Build history of the part. All positions in model axes, mm. Round coordinates to 2 decimals unless told otherwise and drop trailing zeros. Order: outer loops, then holes, each group sorted by start corner. A loop starts at its lowest first (then second) coordinate and runs counter-clockwise, first axis right, second up. Notation, with made-up numbers: M 16,54.25 L 70,54.25 A26 ccw 70,82.25 Z; hole C 87,20.5 d6. An arc over 180 degrees is marked long. Use CSV: the item, a comma, the result in double quotes.
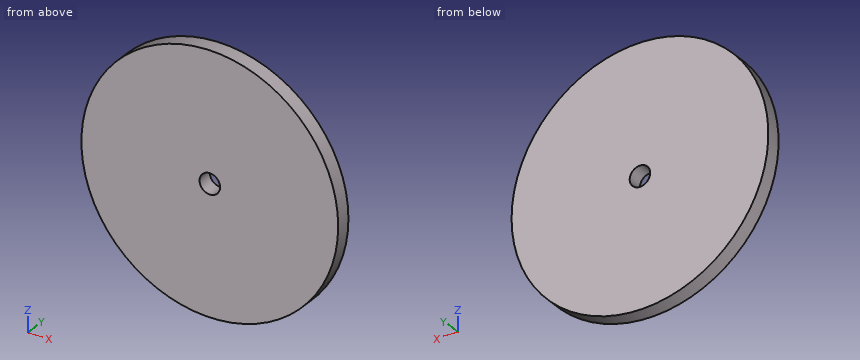
Autodesk Inventor part; units mm, degrees
ref_plane "YZ Plane" through (0, 0, 0) normal (1, 0, 0) x (0, 1, 0)
ref_plane "XZ Plane" through (0, 0, 0) normal (0, 1, 0) x (-1, 0, 0)
ref_plane "XY Plane" through (0, 0, 0) normal (0, 0, 1) x (1, 0, 0)
sketch "スケッチ1" plane through (0, 0, 0) normal (0, 1, 0) x (-1, 0, 0)
  circle A0 centre (0, 0) radius 25
  dimension "d0" = 50
extrude "押し出し1" add sketch "スケッチ1" along normal blind 6
sketch "スケッチ2" plane through (0, 6, 0) normal (0, 1, 0) x (1, 0, 0)
  circle A0 centre (0, 0) radius 4
  dimension "d3" = 8
extrude "押し出し2" cut sketch "スケッチ2" against normal blind 6
sketch "スケッチ3" plane through (0, 0, 0) normal (0, -1, 0) x (1, 0, 0)
  circle A0 centre (0, 0) radius 45
  circle A1 centre (0, 0) radius 4
  circle A2 centre (0, 0) radius 25
  dimension "d6" = 90
  dimension "d7" = 50
extrude "押し出し3" add sketch "スケッチ3" against normal blind 6 contours A0
sketch "スケッチ4" plane through (0, 6, 0) normal (0, 1, 0) x (1, 0, 0)
  circle A0 centre (0, 0) radius 45
  circle A1 centre (0, 0) radius 50
  dimension "d10" = 90
  dimension "d11" = 100
extrude "押し出し4" add sketch "スケッチ4" against normal blind 6
properties part number "NHK_t0_3"
(1) Drop flat-ended pins along their axis: pin 1 (3 mm diameter, centred on x = -20, y = 1.5, fed in from -Z); pin 2 (2 mm diameter, centred on y = 3.5, z = -30, fed in from +X); pin 3 (1.5 mm diameter, centred on x = 14, y = 5, fed in from +Z). Give the stop position or say it passes through.
Answer block:
pin 1,"stops at z = -46.45"
pin 2,"stops at x = 40.73"
pin 3,"stops at z = 48.21"
(2) Cut at B-B, the plane x = 0. Give the cut face in (y, z).
Answer block:
outline,"M 0,-50 L 6,-50 L 6,-4 L 0,-4 Z; M 0,4 L 6,4 L 6,50 L 0,50 Z"
(3) Wall check: line 1 (Z direction, x = 0, y = 2.3); line 2 (X direction, y = 5.5, z = 41.5). Give the ranges that are in metal, low to high. Write a range as from..to.
Answer block:
line 1,"z = -50..-4, 4..50"
line 2,"x = -27.89..27.89"
(4) Cut at A-A, the plane z = 0. Give the cut face in (x, y).
Answer block:
outline,"M -50,0 L -4,0 L -4,6 L -50,6 Z; M 4,0 L 50,0 L 50,6 L 4,6 Z"
(5) Cut at C-C, the plane y = 4.1. Give the cut face in (x, z).
Answer block:
outline,"C 0,0 d100; hole C 0,0 d8"
(6) Cut at D-D, the plane x = 42. Give the cut face in (y, z), and give its area (3 significant figures).
Answer block:
outline,"M 0,-27.13 L 6,-27.13 L 6,27.13 L 0,27.13 Z"
area,"326 mm²"
